Check sheet for the modelled part. Datum: model origin and axes. Units: mm. Face numbers are marked on the shaded views. A direction names the side the tool comes from. Coordinates: 2 decimals unless noted, no trailing zeros. Order: outer loops, then holes, each group sorted by start corner. A loop starts at its lowest first (then second) coordinate and runs counter-clockwise, first axis right, second up.
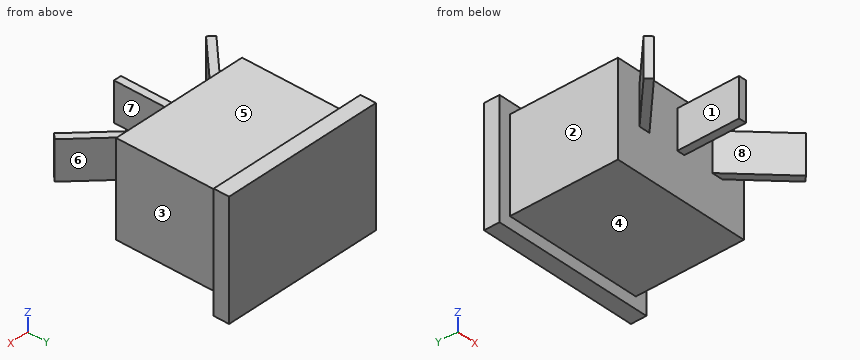
from build123d import *

# Parameters (mm, degrees)
SKETCH1_W                = 18
SKETCH1_H                = 12
BOSS_EXTRUDE1_DEPTH      = 14
SKETCH2_W                = 21
SKETCH2_H                = 15
BOSS_EXTRUDE2_DEPTH      = 2
BOSS_EXTRUDE3_DEPTH      = 2.5
BOSS_EXTRUDE3_DEPTH_BACK = 2.5
SKETCH3_W                = 1
SKETCH3_H                = 8


with BuildPart() as part:
    # Sketch1 → Boss-Extrude1 (new body)
    with BuildSketch(Plane(origin=(0, 0, 0), x_dir=(1, 0, 0), z_dir=(0, 1, 0))):
        with Locations((9, 2)):
            Rectangle(SKETCH1_W, SKETCH1_H)
    extrude(amount=BOSS_EXTRUDE1_DEPTH)

    # Sketch2 → Boss-Extrude2 (add)
    with BuildSketch(Plane(origin=(0, 14, 0), x_dir=(1, 0, 0), z_dir=(0, 1, 0))):
        with Locations((9, 2)):
            Rectangle(SKETCH2_W, SKETCH2_H)
    extrude(amount=BOSS_EXTRUDE2_DEPTH)

    # Sketch3 → Boss-Extrude3 (add, two sides: drawn at the far end of the back side and taken through both)
    with BuildSketch(Plane.XY.offset(-BOSS_EXTRUDE3_DEPTH_BACK)):
        with Locations((9, -4)):
            Rectangle(SKETCH3_W, SKETCH3_H)
        Polygon((13.5, 0), (19.863961031, -6.363961031), (20.571067812, -5.656854249), (14.914213562, 0), align=None)
        Polygon((3.085786438, 0), (4.5, 0), (-1.863961031, -6.363961031), (-2.571067812, -5.656854249), align=None)
    extrude(amount=BOSS_EXTRUDE3_DEPTH + BOSS_EXTRUDE3_DEPTH_BACK)


solid = part.part
(1) Cross-section at A-A (y = -4). Enter the section's corners in (x, z).
Filled in:
outline: (-0.91, -2.5) - (0.5, -2.5) - (0.5, 2.5) - (-0.91, 2.5) - close; (8.5, -2.5) - (9.5, -2.5) - (9.5, 2.5) - (8.5, 2.5) - close; (17.5, -2.5) - (18.91, -2.5) - (18.91, 2.5) - (17.5, 2.5) - close
(2) Tool access check on the marked faces 1, 2, 3, 4 and 5. Record the directions out of +Z, -Z, +X, -X, +Y, -Y that give a thin tool (end or side, any length) a straight path to the whole face; none if there is none.
Filled in:
face 1: +Z, -Z, -Y
face 2: +Z, -Z, -X
face 3: +Z, -Z, +X
face 4: -Z, +X, -X, -Y
face 5: +Z, +X, -X, -Y
(3) Thickness scan on probe 1 along X at (y, z) = (5, -6.25); probe 2 along Y at (x, z) = (7.5, 2); probe 3 along Z at (x, y) = (5, 2.25). Record the ranges inside material, lowest first.
Filled in:
probe 1: x = 0 to 18
probe 2: y = 0 to 16
probe 3: z = -8 to 4
(4) Cross-section at B-B (x = 9). Enter the section's corners in (y, z), and give its area (3 significant figures).
Filled in:
outline: (-8, -2.5) - (0, -2.5) - (0, -8) - (14, -8) - (14, -9.5) - (16, -9.5) - (16, 5.5) - (14, 5.5) - (14, 4) - (0, 4) - (0, 2.5) - (-8, 2.5) - close
area: 238 mm2
(5) Release check for a two-part mould opening along Y. For the marked faces 6, 7 and 8 record: +Y half, -Y half, draft (parallel to the pull), parting line (faces both ways), or undercut.
Filled in:
face 6: undercut
face 7: draft
face 8: -Y half
(6) Cross-section at D-D (y = 14.5). Enter the section's corners in (x, z).
Filled in:
outline: (-1.5, -9.5) - (19.5, -9.5) - (19.5, 5.5) - (-1.5, 5.5) - close
(7) Cross-section at C-C (z = 2). Enter the section's corners in (x, y), and give its area (3 significant figures).
Filled in:
outline: (-2.57, -5.66) - (-1.86, -6.36) - (4.5, 0) - (8.5, 0) - (8.5, -8) - (9.5, -8) - (9.5, 0) - (13.5, 0) - (19.86, -6.36) - (20.57, -5.66) - (14.91, 0) - (18, 0) - (18, 14) - (19.5, 14) - (19.5, 16) - (-1.5, 16) - (-1.5, 14) - (0, 14) - (0, 0) - (3.09, 0) - close
area: 319 mm2
(8) Go/stop test with flat-tipped pins: P1, Ø4, axis at x = 16, y = 2.5, coming from the -Z side; P2, Ø2, axis at y = 15.5, z = -1.5, coming from the -X side; P3, Ø4, axis at y = -3, z = 0.5, coming from the -X side. Record where each tip stops, or that it passes through.
Filled in:
P1: stops at z = -8
P2: stops at x = -1.5
P3: stops at x = -1.91
